Geometry check sheet. Reference: the model listing, model coordinates, mm. Face numbers are marked on the shaded views. A direction names the side the tool comes from. Give positions to 0.01 mm unless a question says otherwise; leave off trailing zeros. Write each loop counter-clockwise with the first axis right and the second up, starting at its lowest first coordinate (ties: lowest second). Pieces come first, ordered by that corner, then holes. Notation, with made-up numbers: (27.25, 5.25) -> (77.25, 5.25) arc R31 ccw to (77.25, 39.25) -> close; hole circle Ø9 at (79.5, 85.25). An arc over 180 degrees is marked (long way). One line per item, written item: value.
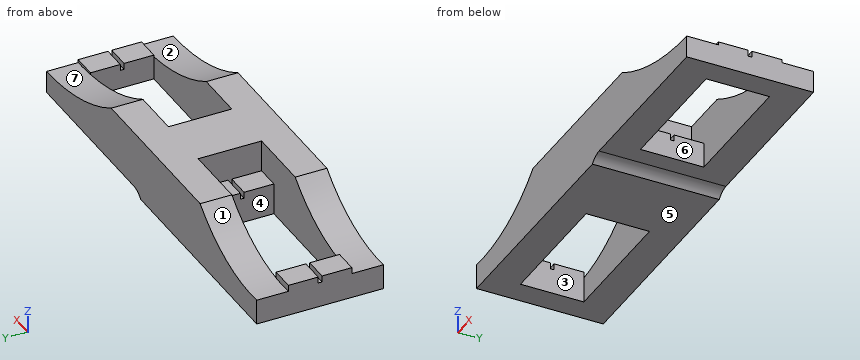
from build123d import *

# Parameters (mm, degrees)
BOSS_EXTRUDE1_DEPTH = 40
SKETCH2_W           = 55.8
SKETCH2_H           = 20
CUT_EXTRUDE1_DEPTH  = 13.5
CUT_EXTRUDE2_REACH  = 79.506
SKETCH3_W           = 40.6
SKETCH3_H           = 20
SKETCH4_W           = 7.6
SKETCH4_H           = 20
BOSS_EXTRUDE2_DEPTH = 3.5
SKETCH5_W           = 55.8
SKETCH5_H           = 1.2
CUT_EXTRUDE3_DEPTH  = 2
SKETCH6_W           = 55.8
SKETCH6_H           = 1.2
CUT_EXTRUDE4_DEPTH  = 2


with BuildPart() as part:
    # Sketch1 → Boss-Extrude1 (new body)
    with BuildSketch(Plane(origin=(0, 0, 0), x_dir=(1, 0, 0), z_dir=(0, 1, 0))):
        with BuildLine():
            Line((65, 8), (23.977973373, 8))
            Line((23.977973373, 8), (10.779053292, 8))
            ThreePointArc((10.779053292, 8), (8.525859954, 8.600007042), (6.661212966, 10))
            Line((6.661212966, 10), (-20, 10))
            Line((-20, 10), (-65, 10))
            Line((-65, 10), (-65, 2))
            ThreePointArc((-65, 2), (-46.256011847, -0.371701222), (-30, -10))
            Line((-30, -10), (-20, -10))
            Line((-20, -10), (17.838709677, -10))
            Line((17.838709677, -10), (20, -10))
            Line((20, -10), (25, -10))
            ThreePointArc((25, -10), (44.283723708, -1.895358938), (65, 1))
            Line((65, 1), (65, 8))
        make_face()
    extrude(amount=BOSS_EXTRUDE1_DEPTH)

    # Sketch2 → Cut-Extrude1 (cut)
    with BuildSketch(Plane.XY.offset(10)):
        with Locations((37.1, 20)):
            Rectangle(SKETCH2_W, SKETCH2_H)
        with Locations((-37.1, 20)):
            Rectangle(SKETCH2_W, SKETCH2_H)
    extrude(amount=-CUT_EXTRUDE1_DEPTH, mode=Mode.SUBTRACT)

    # Sketch3 → Cut-Extrude2 (cut, up to next)
    with BuildSketch(Plane.XY.offset(-3.5), mode=Mode.PRIVATE) as cut_extrude2_sk1:
        with Locations((-37.1, 20)):
            Rectangle(SKETCH3_W, SKETCH3_H)
    cut_extrude2_tool1 = extrude(cut_extrude2_sk1.sketch, amount=-CUT_EXTRUDE2_REACH, mode=Mode.PRIVATE) & part.part
    # Sketch3 → Cut-Extrude2 (cut, up to next)
    with BuildSketch(Plane.XY.offset(-3.5), mode=Mode.PRIVATE) as cut_extrude2_sk2:
        with Locations((37.1, 20)):
            Rectangle(SKETCH3_W, SKETCH3_H)
    cut_extrude2_tool2 = extrude(cut_extrude2_sk2.sketch, amount=-CUT_EXTRUDE2_REACH, mode=Mode.PRIVATE) & part.part
    add(cut_extrude2_tool1.solids().sort_by_distance((-37.1, 20, -3.5))[0], mode=Mode.SUBTRACT)
    add(cut_extrude2_tool2.solids().sort_by_distance((37.1, 20, -3.5))[0], mode=Mode.SUBTRACT)

    # Sketch4 → Boss-Extrude2 (add)
    with BuildSketch(Plane.XY.offset(-3.5)):
        with Locations((-61.2, 20)):
            Rectangle(SKETCH4_W, SKETCH4_H)
        with Locations((-13, 20)):
            Rectangle(SKETCH4_W, SKETCH4_H)
        with Locations((13, 20)):
            Rectangle(SKETCH4_W, SKETCH4_H)
        with Locations((61.2, 20)):
            Rectangle(SKETCH4_W, SKETCH4_H)
    extrude(amount=BOSS_EXTRUDE2_DEPTH)

    # Sketch5 → Cut-Extrude3 (cut)
    with BuildSketch(Plane.XY):
        with Locations((-37.1, 20)):
            Rectangle(SKETCH5_W, SKETCH5_H)
    extrude(amount=-CUT_EXTRUDE3_DEPTH, mode=Mode.SUBTRACT)

    # Sketch6 → Cut-Extrude4 (cut)
    with BuildSketch(Plane.XY):
        with Locations((37.1, 20)):
            Rectangle(SKETCH6_W, SKETCH6_H)
    extrude(amount=-CUT_EXTRUDE4_DEPTH, mode=Mode.SUBTRACT)


solid = part.part
1) Sectioned sample at B-B on x = -46. Record the cut outline in (y, z).
Verdict:
outline: (0, -10) -> (10, -10) -> (10, 0.46) -> (0, 0.46) -> close; (30, -10) -> (40, -10) -> (40, 0.46) -> (30, 0.46) -> close
2) Tool access check on the marked faces 1, 2 and 3. Record the directions out of +Z, -Z, +X, -X, +Y, -Y that give a thin tool (end or side, any length) a straight path to the whole face; none if there is none.
Verdict:
face 1: +Z, +Y
face 2: +Z, +X, -Y
face 3: +Z, -Z
3) Sectioned sample at C-C on z = -4.75. Record the cut outline in (x, y).
Verdict:
outline: (-65, 0) -> (65, 0) -> (65, 40) -> (-65, 40) -> close; hole (-57.4, 10) -> (-16.8, 10) -> (-16.8, 30) -> (-57.4, 30) -> close; hole (16.8, 10) -> (57.4, 10) -> (57.4, 30) -> (16.8, 30) -> close
4) Sectioned sample at A-A on y = 22. Record the cut outline in (x, z), plus the area to 3 significant figures.
Verdict:
outline: (-65, -10) -> (-57.4, -10) -> (-57.4, 0) -> (-65, 0) -> close; (-16.8, -10) -> (6.66, -10) arc R6.11 cw to (10.78, -8) -> (16.8, -8) -> (16.8, 0) -> (9.2, 0) -> (9.2, 10) -> (-9.2, 10) -> (-9.2, 0) -> (-16.8, 0) -> close; (57.4, -8) -> (65, -8) -> (65, 0) -> (57.4, 0) -> close
area: 639 mm^2
5) Depth check by flat-ended pin: pin 1 Ø2.5 at (x, y) = (14.5, 25) entering from +Z; pin 2 Ø0.5 at (x, z) = (62, -0.5) entering from +Y; pin 3 Ø2 at (y, z) = (6.5, 7) entering from +X. Enter the tip coordinate at first touch or a pass-through.
Verdict:
pin 1: z = 0
pin 2: y = 30
pin 3: x = 32.81
6) Scan lines: probe 1 along X at (y, z) = (19, -4.25); probe 2 along Y at (x, z) = (33, -6.75); probe 3 along X at (y, z) = (23, 5). Record each from-to range of solid material in increasing order.
Verdict:
probe 1: -65 to -57.4, -16.8 to 16.8, 57.4 to 65
probe 2: 0 to 10, 30 to 40
probe 3: -9.2 to 9.2
7) Sectioned sample at D-D on y = 32.5. Record the cut outline in (x, z), plus the area to 3 significant figures.
Verdict:
outline: (-65, -10) -> (6.66, -10) arc R6.11 cw to (10.78, -8) -> (65, -8) -> (65, -1) arc R80.99 cw to (25, 10) -> (-30, 10) arc R46.53 cw to (-65, -2) -> close
area: 1,890 mm^2
8) Mould release check, pull along X, two halves, no side actions. Record for the marked faces 4, 5, 6 and 7: released by +X, released by -X, zero draft, split by the parting line, or undercut.
Verdict:
face 4: undercut
face 5: zero draft
face 6: undercut
face 7: released by +X
